CAD build for the part. Positions are in the model's coordinates, mm. A direction names the side the tool comes from. Give positions to 0.01 mm unless a question says otherwise; leave off trailing zeros. Loops run counter-clockwise (first coordinate to the right, second up) from the corner with the lowest first, then second, coordinate; pieces in that order, holes last.
Item 1: Drop flat-ended pins along their axis: P1, Ø1.9, axis at x = 5, y = 0, coming from the -Z side; P2, Ø2, axis at x = -13, z = 1.5, coming from the -Y side; P3, Ø4, axis at x = 6.5, y = 6, coming from the +Z side. Give the stop position or say it passes through.
Item 2: Which spindle directions (+Z, -Z, +X, -X, +Y, -Y) get a long thin tool onto all of the face, cutting with end or side? Do faces 1 (the flat face through (-15, 0, 4.8)), 2 (the flat face through (5.15, 16.87, 0.15)). Say none if no direction does.
Item 3: Probe probe 1 along Z at (x, y) = (16, -7); probe 2 along X at (y, z) = (0.5, 4.3). List the from-to ranges inside material, lowest first.
Item 4: Saw through at C-C on y = -6.5. Give the cut face in (x, z).
Item 5: Mould opens along X. For faces 3 (the cylindrical face through (7.65, -14.04, 0.15)), 4 (the flat face through (0, 1, 0)), 5 (the flat face through (-11.32, -14, 0.15)) say: released by +X, released by -X, zero draft, split by the parting line, or undercut.
Item 6: Saw through at B-B on x = -15. Give the cut face in (y, z).
Item 7: Saw through at A-A on z = 3.65. Give the cut face in (x, y).
from build123d import *

# Parameters (mm, degrees)
F3_DEPTH = 0.3
F4_R     = 1.6
F5_DEPTH = 0.301
F6_R     = 1.5
F7_DEPTH = 4.5
F8_R     = 0.5


with BuildPart() as f3:
    # F2 (on Top) → F3 (new body)
    with BuildSketch(Plane.XY):
        with BuildLine():
            ThreePointArc((22.5701665084, -0.1915041783), (22.6082940696, 0), (22.5701665084, 0.1915041783))
            ThreePointArc((22.5701665084, 0.1915041783), (17.7008675448, 7.675751982), (10.4677268379, 12.9107986006))
            Line((10.4677268379, 12.9107986006), (12.747458202, 15.8287216837))
            Line((12.747458202, 15.8287216837), (12.4964258145, 15.9946956536))
            Line((12.4964258145, 15.9946956536), (10.1887041195, 13.0409465807))
            ThreePointArc((10.1887041195, 13.0409465807), (7.4319060142, 14.1089547165), (4.5662963881, 14.8361813951))
            Line((4.5662963881, 14.8361813951), (5.7490812099, 18.9610422665))
            Line((5.7490812099, 18.9610422665), (5.4607027011, 19.0437334733))
            Line((5.4607027011, 19.0437334733), (4.2698358713, 14.8906872903))
            ThreePointArc((4.2698358713, 14.8906872903), (-0.1360819994, 15.2662877079), (-4.5375427655, 14.8416336361))
            Line((-4.5375427655, 14.8416336361), (-5.7925011179, 18.9464174492))
            Line((-5.7925011179, 18.9464174492), (-6.0793925447, 18.8587059378))
            Line((-6.0793925447, 18.8587059378), (-4.8335659928, 14.7837908983))
            ThreePointArc((-4.8335659928, 14.7837908983), (-7.0006877188, 14.2422664411), (-9.1092972105, 13.5050884949))
            Line((-9.1092972105, 13.5050884949), (-11.2713448253, 16.7104559006))
            Line((-11.2713448253, 16.7104559006), (-11.520056097, 16.5426980296))
            Line((-11.520056097, 16.5426980296), (-9.3929049937, 13.3890668296))
            ThreePointArc((-9.3929049937, 13.3890668296), (-17.2902689379, 8.0970055334), (-22.5701665084, 0.1915041783))
            ThreePointArc((-22.5701665084, 0.1915041783), (-22.6082940696, 0), (-22.5701665084, -0.1915041783))
            ThreePointArc((-22.5701665084, -0.1915041783), (-17.7008675448, -7.675751982), (-10.4677268379, -12.9107986006))
            Line((-10.4677268379, -12.9107986006), (-12.1931284822, -15.1192119975))
            Line((-12.1931284822, -15.1192119975), (-11.9567252562, -15.30391044))
            Line((-11.9567252562, -15.30391044), (-10.1887041195, -13.0409465807))
            ThreePointArc((-10.1887041195, -13.0409465807), (-7.69123576, -14.0245530137), (-5.1009446547, -14.7282729944))
            Line((-5.1009446547, -14.7282729944), (-6.1007225638, -17.8052730061))
            Line((-6.1007225638, -17.8052730061), (-5.8154056089, -17.8979781044))
            Line((-5.8154056089, -17.8979781044), (-4.8053870424, -14.7894605903))
            ThreePointArc((-4.8053870424, -14.7894605903), (0.1368174743, -15.2662836005), (5.0733720825, -14.7341423885))
            Line((5.0733720825, -14.7341423885), (6.1334205771, -17.8127467574))
            Line((6.1334205771, -17.8127467574), (6.4170761498, -17.7150763111))
            Line((6.4170761498, -17.7150763111), (5.3684350935, -14.6696015485))
            ThreePointArc((5.3684350935, -14.6696015485), (7.6806898276, -14.0280478509), (9.9188621728, -13.1627746827))
            Line((9.9188621728, -13.1627746827), (11.6638032097, -15.4783896498))
            Line((11.6638032097, -15.4783896498), (11.9033938627, -15.2978451429))
            Line((11.9033938627, -15.2978451429), (10.1991018341, -13.0361732318))
            ThreePointArc((10.1991018341, -13.0361732318), (17.5983697455, -7.7828218235), (22.5701665084, -0.1915041783))
        make_face()
    extrude(amount=F3_DEPTH)

    # F4 (on face) → F5 (cut, through all)
    with BuildSketch(Plane.XY.offset(0.3)):
        with Locations((5, 0)):
            Circle(F4_R)
        with Locations((-5, 0)):
            Circle(F4_R)
    extrude(amount=-F5_DEPTH, mode=Mode.SUBTRACT)

    # F6 (on face) → F7 (join)
    with BuildSketch(Plane.XY.offset(0.3)):
        with Locations((-15, 0)):
            Circle(F6_R)
        with Locations((15, 0)):
            Circle(F6_R)
    extrude(amount=F7_DEPTH)

    # F8
    f8_edges = [f3.edges().sort_by_distance(p)[0] for p in [
        (-16.5, 0, 4.8),
        (13.5, 0, 4.8),
    ]]
    fillet(f8_edges, radius=F8_R)


solid = f3.part
Results below:
1. P1: passes through
1. P2: stops at y = -1.12
1. P3: stops at z = 0.3
2. face 1: +Z, +X, -X, +Y, -Y
2. face 2: +Z, -Z
3. probe 1: z = 0 to 0.3
3. probe 2: x = -16.41 to -13.59, 13.59 to 16.41
4. outline: (-18.75, 0) - (18.75, 0) - (18.75, 0.3) - (-18.75, 0.3) - close
5. face 3: undercut
5. face 4: zero draft
5. face 5: released by -X
6. outline: (-10.12, 0) - (10.12, 0) - (10.12, 0.3) - (1.5, 0.3) - (1.5, 4.3) arc R0.5 ccw to (1, 4.8) - (-1, 4.8) arc R0.5 ccw to (-1.5, 4.3) - (-1.5, 0.3) - (-10.12, 0.3) - close
7. outline: circle Ø3 at (-15, 0); circle Ø3 at (15, 0)
